Verification items for the finished model (mm, model axes). A direction names the side the tool comes from. Coordinates: 2 decimals unless noted, no trailing zeros. Write each loop counter-clockwise with the first axis right and the second up, starting at its lowest first coordinate (ties: lowest second). Pieces come first, ordered by that corner, then holes. Notation, with made-up numbers: (27, -20) -> (63, -20) arc R23 cw to (63, -3) -> close; hole circle Ø3 at (-13, -5.75). An arc over 180 degrees is marked (long way). Use CSV: the item, a comma, the result in double quotes.
```python
from build123d import *

# Parameters (mm, degrees)
F0_W     = 98
F0_H     = 96
F0_W_2   = 94
F0_H_2   = 92
F1_DEPTH = 10
F0_W_3   = 108
F0_H_3   = 106
F2_DEPTH = 3
F4_D     = 3
F4_DEPTH = 110
F4_START = 5
F4_TIP   = 0.9012909285


with BuildPart() as f1:
    # F0 (on Front) → F1 (new body)
    with BuildSketch(Plane.XZ):
        with Locations((54, 53)):
            Rectangle(F0_W, F0_H)
        with Locations((54, 53)):
            Rectangle(F0_W_2, F0_H_2, mode=Mode.SUBTRACT)
    extrude(amount=F1_DEPTH)

    # F0 (on Front) → F2 (join)
    with BuildSketch(Plane.XZ):
        with Locations((54, 53)):
            Rectangle(F0_W_3, F0_H_3)
        with Locations((54, 53)):
            Rectangle(F0_W, F0_H, mode=Mode.SUBTRACT)
    extrude(amount=F2_DEPTH)

    # F4
    # its depths count from where the whole tool has entered the part; down to there all is cleared
    with Locations(Plane(origin=(0, 0, 0), x_dir=(1, 0, 0), z_dir=(0, 0, -1)).offset(-F4_START)):
        with Locations((12, 5), (96, 5)):
            Hole(F4_D / 2, depth=F4_DEPTH)
            with Locations((0, 0, -(F4_DEPTH + F4_TIP / 2))):  # 118° drill point
                Cone(0, F4_D / 2, F4_TIP, mode=Mode.SUBTRACT)


solid = f1.part
```
1) Cross-section at C-C (x = 96). Record the boundary of the cut face in (y, z).
Return value:
outline,"(-10, 5) -> (-6.5, 5) -> (-6.5, 7) -> (-10, 7) -> close; (-10, 99) -> (-6.5, 99) -> (-6.5, 101) -> (-10, 101) -> close; (-3.5, 5) -> (-3, 5) -> (-3, 0) -> (0, 0) -> (0, 7) -> (-3.5, 7) -> close; (-3.5, 99) -> (0, 99) -> (0, 106) -> (-3, 106) -> (-3, 101) -> (-3.5, 101) -> close"
2) Cross-section at A-A (x = 34). Record the boundary of the cut face in (y, z).
Return value:
outline,"(-10, 5) -> (-3, 5) -> (-3, 0) -> (0, 0) -> (0, 7) -> (-10, 7) -> close; (-10, 99) -> (0, 99) -> (0, 106) -> (-3, 106) -> (-3, 101) -> (-10, 101) -> close"
3) Mould release check, pull along Z, two halves, no side actions. Record for faces 6 (the cylindrical face through (13.5, -5.07, 100.01)), 7 (the flat face through (53, -5, 7)), 8 (the flat face through (53, -1, 0)): released by +Z, released by -Z, zero draft, split by the parting line, or undercut.
Return value:
face 6,"zero draft"
face 7,"undercut"
face 8,"released by -Z"
4) Scan lines: L1, parallel to X at y = -5, z = 100.45; L2, parallel to X at y = -1, z = 77.5; L3, parallel to Z at x = 40, y = -4. Record each from-to range of solid material in increasing order.
Return value:
L1,"5 to 10.5, 13.5 to 94.5, 97.5 to 103"
L2,"0 to 7, 101 to 108"
L3,"5 to 7, 99 to 101"
5) Set-up check for faces 1 (the flat face through (101, -5, 52)), 2 (the flat face through (53, -1, 106)), 3 (the flat face through (103, -6, 52)), 4 (the flat face through (5, -6, 52)), 5 (the flat face through (53, -6, 101)): record each of +Z, -Z, +X, -X, +Y, -Y from which the full face is reachable in a straight line by a thin tool's end or side.
Return value:
face 1,"+Y, -Y"
face 2,"+Z, +X, -X, +Y, -Y"
face 3,"+Z, -Z, +X, -Y"
face 4,"+Z, -Z, -X, -Y"
face 5,"+Z, +X, -X, -Y"
6) Gauge pin test, flat ends, axial feed: pin 1 (6 mm diameter, centred on x = 35, y = -2, fed in from -Z); pin 2 (5 mm diameter, centred on x = 74.5, y = -6.5, fed in from +Z); pin 3 (4 mm diameter, centred on y = -6, z = 24.5, fed in from -X); pin 4 (3.5 mm diameter, centred on x = 12, y = -5, fed in from -Z). Record the tip position at first contact, or that the pin passes through.
Return value:
pin 1,"z = 0"
pin 2,"z = 101"
pin 3,"x = 5"
pin 4,"z = 5"
7) Cross-section at B-B (z = 96.5). Record the boundary of the cut face in (x, y), plus the area to 3 significant figures.
Return value:
outline,"(0, -3) -> (5, -3) -> (5, -10) -> (7, -10) -> (7, 0) -> (0, 0) -> close; (101, -10) -> (103, -10) -> (103, -3) -> (108, -3) -> (108, 0) -> (101, 0) -> close"
area,"70.0 mm2"
8) Cross-section at D-D (y = -5). Record the boundary of the cut face in (x, z), plus the area to 3 significant figures.
Return value:
outline,"(5, 5) -> (10.5, 5) -> (10.5, 7) -> (7, 7) -> (7, 99) -> (10.5, 99) -> (10.5, 101) -> (5, 101) -> close; (13.5, 5) -> (94.5, 5) -> (94.5, 7) -> (13.5, 7) -> close; (13.5, 99) -> (94.5, 99) -> (94.5, 101) -> (13.5, 101) -> close; (97.5, 5) -> (103, 5) -> (103, 101) -> (97.5, 101) -> (97.5, 99) -> (101, 99) -> (101, 7) -> (97.5, 7) -> close"
area,"736 mm2"
